Design review of the part shown in the three views and the two pictorial views. Dimensions are in mm from the part's minimum x, y and z. Give positions to 0.01 mm unless a question says otherwise; leave off trailing zeros. Write each loop counter-clockwise with the first axis right and the second up, starting at its lowest first coordinate (ties: lowest second). Pieces come first, ordered by that corner, then holes. Notation, with made-up numbers: (13.25, 37.5) -> (18.25, 37.5) arc R21 ccw to (18.25, 51.5) -> close; hole circle Ø8 at (0.25, -29.5). An arc over 180 degrees is marked (long way). Return JSON: item names as keys, results as strings. Group by question number.
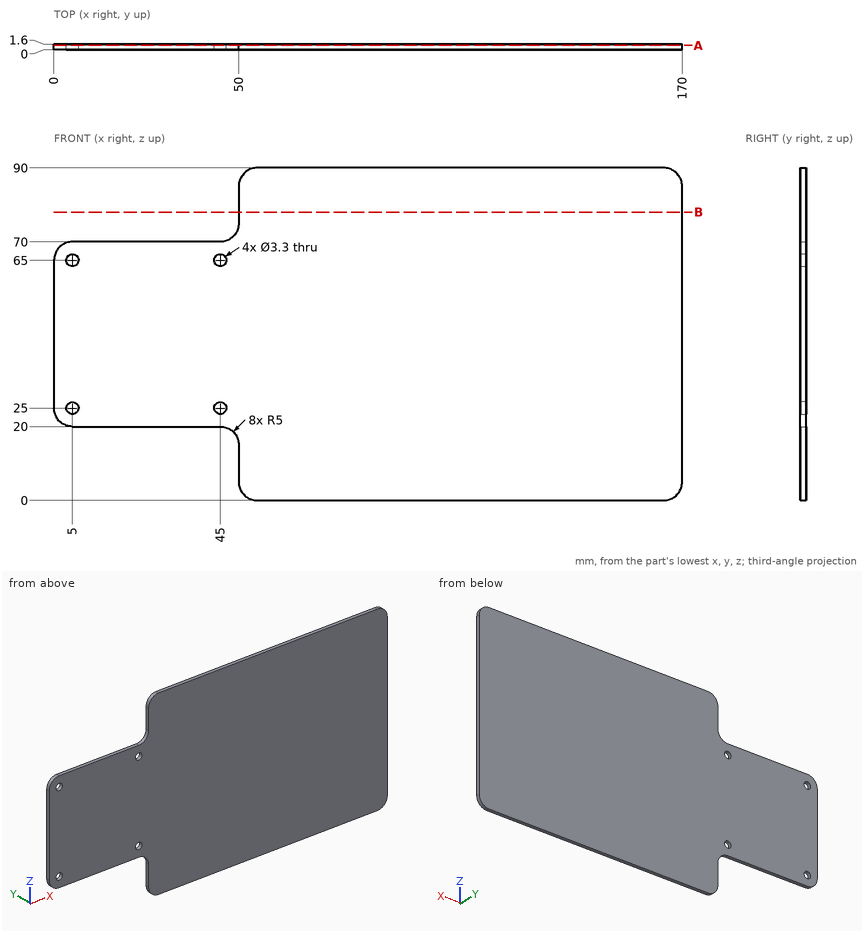
Q1. Take a section at A-A, the plane y = 1.25. Give the boundary of the cut face in (x, z).
Q2. Insertion check: pin 1 (0.5 mm diameter, centred on y = 1, z = 78, fed in from -X); pin 2 (0.8 mm diameter, centred on x = 31.5, y = 0.5, fed in from -Z); pin 3 (4 mm diameter, centred on x = 5, z = 25, fed in from +Y); pin 4 (2 mm diameter, centred on x = 45, z = 65, fed in from +Y). Each pin has a flat end and moves straight along its axis. Give the tip position at first contact, or say it passes through.
Q3. For L1, parallel to X at y = 1.15, z = 25; L2, parallel to Z at x = 13.5, y = 1.35; L3, parallel to Z at x = 47, y = 1.1, list the stretches that pass through material, from the lowest coordinate up. Write a range as from..to.
Q4. Take a section at B-B, the plane z = 78. Give the boundary of the cut face in (x, y).
Final values:
{
 "1": {"outline": "(0, 25) arc R5 ccw to (5, 20) -> (45, 20) arc R5 cw to (50, 15) -> (50, 5) arc R5 ccw to (55, 0) -> (165, 0) arc R5 ccw to (170, 5) -> (170, 85) arc R5 ccw to (165, 90) -> (55, 90) arc R5 ccw to (50, 85) -> (50, 75) arc R5 cw to (45, 70) -> (5, 70) arc R5 ccw to (0, 65) -> close; hole circle Ø3.3 at (5, 25); hole circle Ø3.3 at (5, 65); hole circle Ø3.3 at (45, 25); hole circle Ø3.3 at (45, 65)"},
 "2": {"pin 1": "stops at x = 50", "pin 2": "stops at z = 20", "pin 3": "stops at y = 1.6", "pin 4": "passes through"},
 "3": {"L1": "x = 0..3.35, 6.65..43.35, 46.65..170", "L2": "z = 20..70", "L3": "z = 19.58..70.42"},
 "4": {"outline": "(50, 0) -> (170, 0) -> (170, 1.6) -> (50, 1.6) -> close"}
}
